```python
from build123d import *

# Parameters (mm, degrees)
SKETCH_1_W          = 25
SKETCH_1_H          = 30
EXTRUDE_1_DEPTH     = 1.5
SKETCH_2_R          = 1.5
CUT_EXTRUDE_1_DEPTH = 21.5
EXTRUDE_2_DEPTH     = 3
FILLET_1_R          = 2
SKETCH_4_R          = 7.5
CUT_EXTRUDE_2_DEPTH = 10


with BuildPart() as part:
    # 草图1 → 凸台-拉伸1 (new, symmetric)
    with BuildSketch(Plane.XY):
        with Locations((12.5, -15)):
            Rectangle(SKETCH_1_W, SKETCH_1_H)
        Polygon((0, 25), (0, 0), (25, 0), (55, 0), (55, 25), align=None)
    extrude(amount=EXTRUDE_1_DEPTH, both=True)

    # 草图2 → 切除-拉伸1 (cut, symmetric)
    with BuildSketch(Plane.XY.offset(1.5)):
        with Locations((20, -25)):
            Circle(SKETCH_2_R)
        with Locations((5, -25)):
            Circle(SKETCH_2_R)
        with Locations((5, -5)):
            Circle(SKETCH_2_R)
        with Locations((20, -5)):
            Circle(SKETCH_2_R)
        with Locations((30, 5)):
            Circle(SKETCH_2_R)
        with Locations((30, 20)):
            Circle(SKETCH_2_R)
        with Locations((50, 20)):
            Circle(SKETCH_2_R)
        with Locations((50, 5)):
            Circle(SKETCH_2_R)
    extrude(amount=CUT_EXTRUDE_1_DEPTH, both=True, mode=Mode.SUBTRACT)

    # 草图3 → 凸台-拉伸2 (add)
    with BuildSketch(Plane.XY.offset(1.5)):
        Polygon((25, -5.656854249), (30.656854249, 0), (25, 0), align=None)
    extrude(amount=-EXTRUDE_2_DEPTH)

    # 圆角1
    fillet_1_edges = [part.edges().sort_by_distance(p)[0] for p in [
        (25, -30, 0),
        (0, -30, 0),
        (0, 25, 0),
        (55, 25, 0),
        (55, 0, 0),
        (25, -5.656854249, 0),
        (30.656854249, 0, 0),
    ]]
    fillet(fillet_1_edges, radius=FILLET_1_R)

    # 草图4 → 切除-拉伸2 (cut)
    with BuildSketch(Plane.XY.offset(1.5)):
        with Locations((12.5, 12.5)):
            Circle(SKETCH_4_R)
    extrude(amount=-CUT_EXTRUDE_2_DEPTH, mode=Mode.SUBTRACT)


solid = part.part
```
Check sheet for the modelled part. Datum: model origin and axes. Units: mm. A direction names the side the tool comes from. Give positions to 0.01 mm unless a question says otherwise; leave off trailing zeros. Order: outer loops, then holes, each group sorted by start corner. A loop starts at its lowest first (then second) coordinate and runs counter-clockwise, first axis right, second up. Notation, with made-up numbers: M 37.25,56 L 64.25,56 A17 cw 64.25,73 Z; hole C 50,-34.5 d1. An arc over 180 degrees is marked long. Answer in a Markdown table with one row per item. Add a question column.
Q1. Access from +Z, -Z, +X, -X, +Y, -Y to the whole of each face (thin tool, end or side, straight path). Record for faces 1 (the flat face through (42, 0, 0)), 2 (the flat face through (12, -30, 0)).
Q2. Gauge pin test, flat ends, axial feed: pin 1 Ø1 at (x, z) = (47.5, 1) entering from -Y; pin 2 Ø1.5 at (y, z) = (-20, -0.5) entering from +X. Record the tip position at first contact, or that the pin passes through.
Q3. Sectioned sample at B-B, the plane z = 0.6. Count the separate pieces of the cut face and the enclosed holes in it, and give its area (3 significant figures).
Q4. Thickness scan on L1, parallel to Y at x = 30, z = 0.3; L2, parallel to Y at x = 12.5, z = 0.4; L3, parallel to X at y = -15, z = 0.95. Record the ranges inside material, lowest first.
Q5. Release check for a two-part mould opening along X. For faces 3 (the cylindrical face through (30.71, -0.156, -0.021)), 4 (the cylindrical face through (5.806, -3.735, 0.021)), 5 (the cylindrical face through (18.89, -23.99, 0.02)), 6 (the flat face through (0, -2, 0)) record: released by +X, released by -X, zero draft, split by the parting line, or undercut.
Q6. Sectioned sample at C-C, the plane y = 12.5. Record the boundary of the cut face in (x, z).
Q7. Sectioned sample at A-A, the plane x = 50. Record the boundary of the cut face in (y, z), and give its area (3 significant figures).
Verdict:
| question | item | result |
|---|---|---|
| 1 | face 1 | +Z, -Z, +X, -Y |
| 1 | face 2 | +Z, -Z, +X, -X, -Y |
| 2 | pin 1 | y = 0 |
| 2 | pin 2 | x = 25 |
| 3 | separate pieces | 1 |
| 3 | enclosed holes | 9 |
| 3 | area | 1,900 mm² |
| 4 | L1 | -0.66 to 3.5, 6.5 to 18.5, 21.5 to 25 |
| 4 | L2 | -30 to 5, 20 to 25 |
| 4 | L3 | 0 to 25 |
| 5 | face 3 | released by +X |
| 5 | face 4 | undercut |
| 5 | face 5 | undercut |
| 5 | face 6 | released by -X |
| 6 | outline | M 0,-1.5 L 5,-1.5 L 5,1.5 L 0,1.5 Z; M 20,-1.5 L 55,-1.5 L 55,1.5 L 20,1.5 Z |
| 7 | outline | M 0,-1.5 L 3.5,-1.5 L 3.5,1.5 L 0,1.5 Z; M 6.5,-1.5 L 18.5,-1.5 L 18.5,1.5 L 6.5,1.5 Z; M 21.5,-1.5 L 25,-1.5 L 25,1.5 L 21.5,1.5 Z |
| 7 | area | 57.0 mm² |
